Part print with two shaded views. Sizes in mm from the minimum x, y, z corner. Round coordinates to 2 decimals unless told otherwise and drop trailing zeros. Write each loop counter-clockwise with the first axis right and the second up, starting at its lowest first coordinate (ties: lowest second). Pieces come first, ordered by that corner, then holes. Notation, with made-up numbers: (2.5, 63.5) -> (44.5, 63.5) arc R27 cw to (44.5, 87.5) -> close; hole circle Ø1 at (-35, 28). An arc over 180 degrees is marked (long way). Return JSON: item names as keys, results as strings. Group by question number.
(1) Drill centre lines: L1, parallel to Z at x = 22, y = 4.25; L2, parallel to Z at x = 31.75, y = 3; L3, parallel to X at y = 1, z = 6.5. Where is each one in solid material? Low to high. Write a range as from..to.
(2) Saw through at A-A (z = 107.95). List the corners of the cut face in (x, y).
(3) Saw through at B-B (x = 31.75). List the corners of the cut face in (y, z).
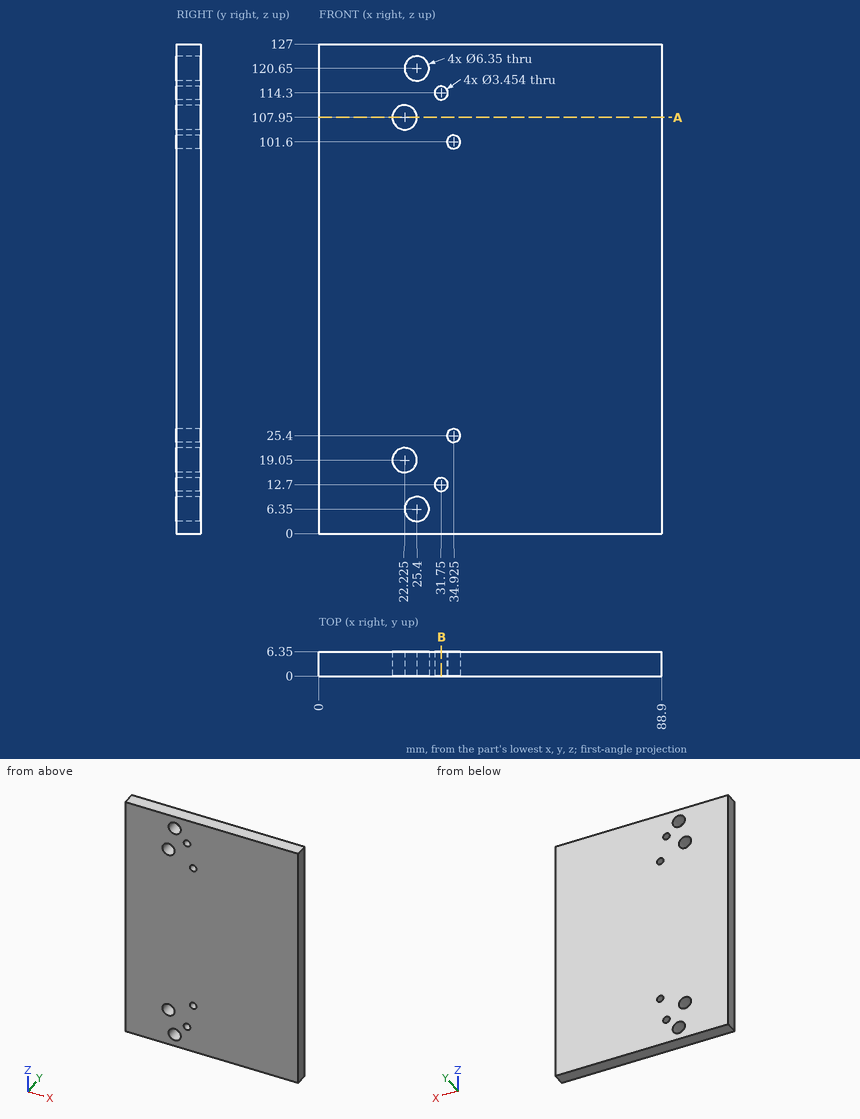
Computed values:
{
 "1": {"L1": "0..15.88, 22.22..104.78, 111.12..127", "L2": "0..10.97, 14.43..112.57, 116.03..127", "L3": "0..22.23, 28.57..88.9"},
 "2": {"outline": "(0, 0) -> (19.05, 0) -> (19.05, 6.35) -> (0, 6.35) -> close; (25.4, 0) -> (88.9, 0) -> (88.9, 6.35) -> (25.4, 6.35) -> close"},
 "3": {"outline": "(0, 0) -> (6.35, 0) -> (6.35, 10.97) -> (0, 10.97) -> close; (0, 14.43) -> (6.35, 14.43) -> (6.35, 112.57) -> (0, 112.57) -> close; (0, 116.03) -> (6.35, 116.03) -> (6.35, 127) -> (0, 127) -> close"}
}
